Verification items for the finished model (mm, model axes). Face numbers are marked on the shaded views. A direction names the side the tool comes from. Coordinates: 2 decimals unless noted, no trailing zeros. Write each loop counter-clockwise with the first axis right and the second up, starting at its lowest first coordinate (ties: lowest second). Pieces come first, ordered by that corner, then holes. Notation, with made-up numbers: (10.5, -40) -> (52.5, -40) arc R32 cw to (52.5, -5) -> close; hole circle Ø8 at (-33.75, -29). An arc over 180 degrees is marked (long way). Answer in a Markdown table with one row per item.
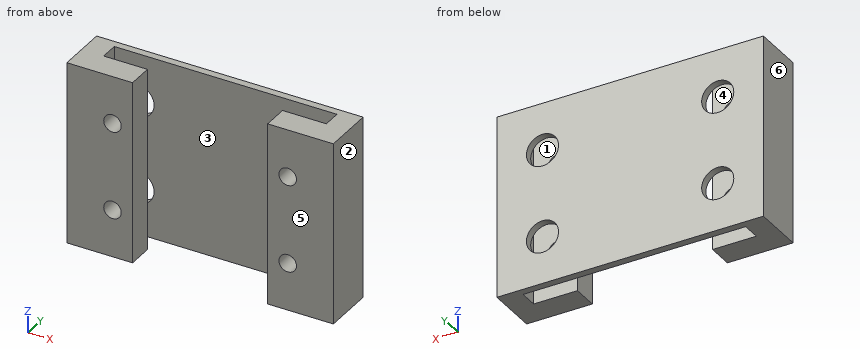
```python
from build123d import *

# Parameters (mm, degrees)
EXTRUDE_3_DEPTH             = 12.5
HOLE_WIZARD_M21_D           = 2.4
HOLE_WIZARD_M21_CSINK_D     = 4.4
HOLE_WIZARD_M21_CSINK_ANGLE = 90
CUT_EXTRUDE_1_REACH         = 25.202
SKETCH_6_R                  = 2.2


with BuildPart() as part:
    # Эскиз3 → Бобышка-Вытянуть3 (new, symmetric)
    with BuildSketch(Plane.XY):
        Polygon((-9.25, 0), (-18.25, 0), (-18.25, 7), (18.25, 7), (18.25, 0), (9.25, 0), (9.25, 3.5), (15.25, 3.5), (15.25, 6), (-15.25, 6), (-15.25, 3.5), (-9.25, 3.5), align=None)
    extrude(amount=EXTRUDE_3_DEPTH, both=True)

    # Зенковка для винта с потайной головкой M21 (through all)
    with Locations(Plane(origin=(0, 7, 0), x_dir=(1, 0, 0), z_dir=(0, 1, 0))):
        with Locations((-12, 6), (-12, -6), (12, -6), (12, 6)):
            CounterSinkHole(HOLE_WIZARD_M21_D / 2, HOLE_WIZARD_M21_CSINK_D / 2, counter_sink_angle=HOLE_WIZARD_M21_CSINK_ANGLE)

    # Эскиз6 → Вырез-Вытянуть1 (cut, up to next)
    with BuildSketch(Plane(origin=(0, 7, 0), x_dir=(1, 0, 0), z_dir=(0, 1, 0)), mode=Mode.PRIVATE) as cut_extrude_1_sk1:
        with Locations(Location((-12, -6, 0), (0, 0, 180))):
            Circle(SKETCH_6_R)
    cut_extrude_1_tool1 = extrude(cut_extrude_1_sk1.sketch, amount=-CUT_EXTRUDE_1_REACH, mode=Mode.PRIVATE) & part.part
    # Эскиз6 → Вырез-Вытянуть1 (cut, up to next)
    with BuildSketch(Plane(origin=(0, 7, 0), x_dir=(1, 0, 0), z_dir=(0, 1, 0)), mode=Mode.PRIVATE) as cut_extrude_1_sk2:
        with Locations(Location((12, -6, 0), (0, 0, 180))):
            Circle(SKETCH_6_R)
    cut_extrude_1_tool2 = extrude(cut_extrude_1_sk2.sketch, amount=-CUT_EXTRUDE_1_REACH, mode=Mode.PRIVATE) & part.part
    # Эскиз6 → Вырез-Вытянуть1 (cut, up to next)
    with BuildSketch(Plane(origin=(0, 7, 0), x_dir=(1, 0, 0), z_dir=(0, 1, 0)), mode=Mode.PRIVATE) as cut_extrude_1_sk3:
        with Locations(Location((12, 6, 0), (0, 0, 180))):
            Circle(SKETCH_6_R)
    cut_extrude_1_tool3 = extrude(cut_extrude_1_sk3.sketch, amount=-CUT_EXTRUDE_1_REACH, mode=Mode.PRIVATE) & part.part
    # Эскиз6 → Вырез-Вытянуть1 (cut, up to next)
    with BuildSketch(Plane(origin=(0, 7, 0), x_dir=(1, 0, 0), z_dir=(0, 1, 0)), mode=Mode.PRIVATE) as cut_extrude_1_sk4:
        with Locations(Location((-12, 6, 0), (0, 0, 180))):
            Circle(SKETCH_6_R)
    cut_extrude_1_tool4 = extrude(cut_extrude_1_sk4.sketch, amount=-CUT_EXTRUDE_1_REACH, mode=Mode.PRIVATE) & part.part
    add(cut_extrude_1_tool1.solids().sort_by_distance((-12, 7, 6))[0], mode=Mode.SUBTRACT)
    add(cut_extrude_1_tool2.solids().sort_by_distance((12, 7, 6))[0], mode=Mode.SUBTRACT)
    add(cut_extrude_1_tool3.solids().sort_by_distance((12, 7, -6))[0], mode=Mode.SUBTRACT)
    add(cut_extrude_1_tool4.solids().sort_by_distance((-12, 7, -6))[0], mode=Mode.SUBTRACT)


solid = part.part
```
1. Sectioned sample at D-D, the plane y = 4. Record the cut outline in (x, z).
Findings below:
| item | result |
|---|---|
| outline | (-18.25, -12.5) -> (-15.25, -12.5) -> (-15.25, 12.5) -> (-18.25, 12.5) -> close; (15.25, -12.5) -> (18.25, -12.5) -> (18.25, 12.5) -> (15.25, 12.5) -> close |
2. Go/stop test with a flat-tipped pin: pin 1 (2 mm diameter, centred on x = -11.5, z = -6, fed in from +Y). Record where the tip stops, or that it passes through.
Findings below:
| item | result |
|---|---|
| pin 1 | stops at y = 3.5 |
3. Sectioned sample at A-A, the plane y = 1.5. Record the cut outline in (x, z).
Findings below:
| item | result |
|---|---|
| outline | (-18.25, -12.5) -> (-9.25, -12.5) -> (-9.25, 12.5) -> (-18.25, 12.5) -> close; (9.25, -12.5) -> (18.25, -12.5) -> (18.25, 12.5) -> (9.25, 12.5) -> close; hole circle Ø2.4 at (-12, -6); hole circle Ø2.4 at (-12, 6); hole circle Ø2.4 at (12, -6); hole circle Ø2.4 at (12, 6) |
4. Release check for a two-part mould opening along Y. For the marked faces 3, 4, 5 and 6 record: released by +Y, released by -Y, zero draft, split by the parting line, or undercut.
Findings below:
| item | result |
|---|---|
| face 3 | undercut |
| face 4 | undercut |
| face 5 | released by -Y |
| face 6 | zero draft |
5. Sectioned sample at C-C, the plane z = 6. Record the cut outline in (x, y), and give its area (3 significant figures).
Findings below:
| item | result |
|---|---|
| outline | (-18.25, 0) -> (-13.2, 0) -> (-13.2, 3.5) -> (-15.25, 3.5) -> (-15.25, 6) -> (-14.2, 6) -> (-14.2, 7) -> (-18.25, 7) -> close; (-10.8, 0) -> (-9.25, 0) -> (-9.25, 3.5) -> (-10.8, 3.5) -> close; (-9.8, 6) -> (9.8, 6) -> (9.8, 7) -> (-9.8, 7) -> close; (9.25, 0) -> (10.8, 0) -> (10.8, 3.5) -> (9.25, 3.5) -> close; (13.2, 0) -> (18.25, 0) -> (18.25, 7) -> (14.2, 7) -> (14.2, 6) -> (15.25, 6) -> (15.25, 3.5) -> (13.2, 3.5) -> close |
| area | 88.9 mm² |
6. Sectioned sample at B-B, the plane x = -12. Record the cut outline in (y, z), and give its area (3 significant figures).
Findings below:
| item | result |
|---|---|
| outline | (0, -12.5) -> (3.5, -12.5) -> (3.5, -7.2) -> (0, -7.2) -> close; (0, -4.8) -> (3.5, -4.8) -> (3.5, 4.8) -> (0, 4.8) -> close; (0, 7.2) -> (3.5, 7.2) -> (3.5, 12.5) -> (0, 12.5) -> close; (6, -12.5) -> (7, -12.5) -> (7, -8.2) -> (6, -8.2) -> close; (6, -3.8) -> (7, -3.8) -> (7, 3.8) -> (6, 3.8) -> close; (6, 8.2) -> (7, 8.2) -> (7, 12.5) -> (6, 12.5) -> close |
| area | 86.9 mm² |
7. Access from +Z, -Z, +X, -X, +Y, -Y to the whole of each face (thin tool, end or side, straight path). Record for the marked faces 1 and 2.
Findings below:
| item | result |
|---|---|
| face 1 | +Z, -Z |
| face 2 | +Z, -Z, +X, +Y, -Y |
8. Material ranges on probe 1 along Z at (x, y) = (12, 2.75); probe 2 along X at (y, z) = (6.45, 6); probe 3 along X at (y, z) = (1.5, -6), recorded low to high. Write a range as from..to.
Findings below:
| item | result |
|---|---|
| probe 1 | z = -12.5..-7.2, -4.8..4.8, 7.2..12.5 |
| probe 2 | x = -18.25..-14.2, -9.8..9.8, 14.2..18.25 |
| probe 3 | x = -18.25..-13.2, -10.8..-9.25, 9.25..10.8, 13.2..18.25 |
